CAD build for the part. Positions are in the model's coordinates, mm. Give positions to 0.01 mm unless a question says otherwise; leave off trailing zeros. Order: outer loops, then holes, each group sorted by start corner. A loop starts at its lowest first (then second) coordinate and runs counter-clockwise, first axis right, second up. Notation, with made-up numbers: M -34.5,6.5 L 20.5,6.5 A8 cw 20.5,12.5 Z; hole C 24,-15.5 d9. An arc over 180 degrees is marked long. Put each result on its own line as item: value. Start each with the question number.
1) Cut at C-C (x = 4). Write the cut outline in (y, z), and give its area (3 significant figures).
2) Cut at B-B (z = 0.35). Write the cut outline in (x, y).
3) Cut at D-D (x = -3.75). Write the cut outline in (y, z), and give its area (3 significant figures).
4) Cut at A-A (x = 0). Write the cut outline in (y, z).
5) Drill centre lines: line 1 (Y direction, x = 0.25, z = -0.35); line 2 (X direction, y = -3.5, z = 0.7); line 3 (Y direction, x = -0.5, z = 0.65). Where is each one in solid material? Low to high. Write a range as [from, to].
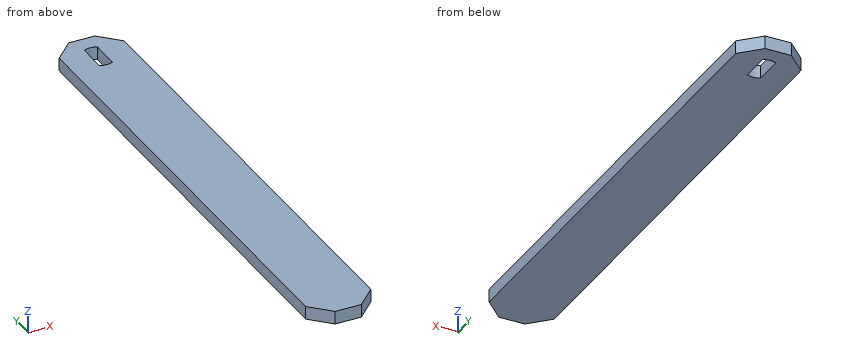
```python
from build123d import *

# Parameters (mm, degrees)
F0_W     = 10
F0_H     = 2
F1_DEPTH = 80
F3_DEPTH = 2
F4_SIZE  = 3


with BuildPart() as f1:
    # F0 (on Front) → F1 (new body)
    with BuildSketch(Plane.XZ):
        Rectangle(F0_W, F0_H)
    extrude(amount=F1_DEPTH)

    # F2 (on face) → F3 (cut, through all)
    with BuildSketch(Plane.XY.offset(1)):
        with BuildLine():
            Line((1, -7.291288), (1, -2.708712))
            ThreePointArc((1, -2.708712), (0, -2.5), (-1, -2.708712))
            Line((-1, -2.708712), (-1, -7.291288))
            ThreePointArc((-1, -7.291288), (0, -7.5), (1, -7.291288))
        make_face()
    extrude(amount=-F3_DEPTH, mode=Mode.SUBTRACT)

    # F4
    f4_edges = [f1.edges().sort_by_distance(p)[0] for p in [
        (-5, 0, 0),
        (5, 0, 0),
        (-5, -80, 0),
        (5, -80, 0),
    ]]
    chamfer(f4_edges, length=F4_SIZE)


solid = f1.part
```
Solution:
1. outline: M -78,-1 L -2,-1 L -2,1 L -78,1 Z
1. area: 152 mm²
2. outline: M -5,-77 L -2,-80 L 2,-80 L 5,-77 L 5,-3 L 2,0 L -2,0 L -5,-3 Z; hole M -1,-7.29 A2.5 ccw 1,-7.29 L 1,-2.71 A2.5 ccw -1,-2.71 Z
3. outline: M -78.25,-1 L -1.75,-1 L -1.75,1 L -78.25,1 Z
3. area: 153 mm²
4. outline: M -80,-1 L -7.5,-1 L -7.5,1 L -80,1 Z; M -2.5,-1 L 0,-1 L 0,1 L -2.5,1 Z
5. line 1: [-80, -7.49], [-2.51, 0]
5. line 2: [-5, -1], [1, 5]
5. line 3: [-80, -7.45], [-2.55, 0]
